Part model, mm, in its own coordinate system. A direction names the side the tool comes from. Round coordinates to 2 decimals unless told otherwise and drop trailing zeros. Loops run counter-clockwise (first coordinate to the right, second up) from the corner with the lowest first, then second, coordinate; pieces in that order, holes last.
1) Band-saw the part on A-A, the plane x = 0. Write the cut outline in (y, z), then the cut area to 3 significant figures.
2) Band-saw the part on B-B, the plane z = -1.5. Write the cut outline in (x, y), then the cut area to 3 significant figures.
3) Band-saw the part on C-C, the plane y = -17.25. Write the cut outline in (x, z), then the cut area to 3 significant figures.
4) 3-axis set-ups, long thin cutter, end or side, ignore diameter. For faces 1 (the flat face through (-21, 0, 15)), 2 (the cylindrical face through (-8.771, -12.325, 44.218)): which of +Z, -Z, +X, -X, +Y, -Y reach the whole face in a straight line?
5) Probe line 1 (Z direction, x = 0, y = -10.5); line 2 (X direction, y = -19, z = 29.5); line 3 (X direction, y = -18.25, z = 30). List the from-to ranges inside material, lowest first.
6) Drop flat-ended pins along their axis: P1, Ø6, axis at x = -23, y = -22.5, coming from the -Z side; P2, Ø10, axis at x = 24.94, z = 42.32, coming from the -Y side; P3, Ø1.5, axis at x = 19, z = 33, coming from the +Y side; P4, Ø2, axis at x = -32, y = -9, coming from the -Z side. Give the stop position or say it passes through.
from build123d import *

# Parameters (mm, degrees)
F0_R     = 5.194766
F0_R_2   = 8.44897
F0_R_3   = 5.580151
F1_DEPTH = 25


with BuildPart() as f1:
    # F0 (on Front) → F1 (new body)
    with BuildSketch(Plane.XZ):
        with BuildLine():
            ThreePointArc((-42.153431, 15.49969), (-22.537107, 7.573578), (-7.372486, -7.17965))
            ThreePointArc((-7.372486, -7.17965), (0.675671, -10.268612), (8.249685, -6.151716))
            Line((8.249685, -6.151716), (33.641666, 37.229096))
            ThreePointArc((33.641666, 37.229096), (34.332195, 45.988125), (27.889637, 51.962307))
            ThreePointArc((27.889637, 51.962307), (26.800193, 52.173359), (25.708755, 52.373848))
            ThreePointArc((25.708755, 52.373848), (-10.031283, 53.094379), (-44.25329, 42.76366))
            ThreePointArc((-44.25329, 42.76366), (-44.294203, 42.743895), (-44.335109, 42.724113))
            ThreePointArc((-44.335109, 42.724113), (-55.303805, 29.696455), (-45.187778, 15.996156))
            ThreePointArc((-45.187778, 15.996156), (-43.746778, 15.782133), (-42.311961, 15.529965))
            ThreePointArc((-42.311961, 15.529965), (-42.232685, 15.514886), (-42.153431, 15.49969))
        make_face()
        Circle(F0_R, mode=Mode.SUBTRACT)
        with Locations((-41.56223, 29.258074)):
            Circle(F0_R_2, mode=Mode.SUBTRACT)
        with BuildLine():
            Line((19.861759, 33.613489), (5.336992, 8.798718))
            ThreePointArc((5.336992, 8.798718), (0.233138, 10.288176), (-4.932946, 9.031443))
            ThreePointArc((-4.932946, 9.031443), (-15.984396, 17.984335), (-28.67212, 24.411659))
            ThreePointArc((-28.67212, 24.411659), (-27.982255, 31.544326), (-30.969534, 38.057929))
            ThreePointArc((-30.969534, 38.057929), (-8.443879, 44.251791), (14.867818, 42.724113))
            ThreePointArc((14.867818, 42.724113), (16.100782, 37.475942), (19.861759, 33.613489))
        make_face(mode=Mode.SUBTRACT)
        with Locations((24.941154, 42.321745)):
            Circle(F0_R_3, mode=Mode.SUBTRACT)
        with BuildLine():
            ThreePointArc((-44.25329, 42.76366), (-55.292646, 28.200564), (-42.153431, 15.49969))
            ThreePointArc((-42.153431, 15.49969), (-42.232685, 15.514886), (-42.311961, 15.529965))
            ThreePointArc((-42.311961, 15.529965), (-43.762253, 15.686672), (-45.187778, 15.996156))
            ThreePointArc((-45.187778, 15.996156), (-55.303805, 29.696455), (-44.335109, 42.724113))
            ThreePointArc((-44.335109, 42.724113), (-44.294203, 42.743895), (-44.25329, 42.76366))
        make_face()
        with BuildLine():
            ThreePointArc((25.708755, 52.373848), (26.800193, 52.173359), (27.889637, 51.962307))
            ThreePointArc((27.889637, 51.962307), (26.810555, 52.228274), (25.708755, 52.373848))
        make_face()
    extrude(amount=F1_DEPTH)


solid = f1.part
Reported:
1. outline: (-25, -10.29) - (0, -10.29) - (0, -5.19) - (-25, -5.19) - close; (-25, 5.19) - (0, 5.19) - (0, 10.29) - (-25, 10.29) - close; (-25, 44.6) - (0, 44.6) - (0, 54.03) - (-25, 54.03) - close
1. area: 490 mm2
2. outline: (-11.89, -25) - (-4.97, -25) - (-4.97, 0) - (-11.89, 0) - close; (4.97, -25) - (10.97, -25) - (10.97, 0) - (4.97, 0) - close
2. area: 323 mm2
3. outline: (-44.25, 42.76) arc R13.77 ccw to (-42.15, 15.5) arc R54.92 cw to (-7.37, -7.18) arc R10.29 ccw to (8.25, -6.15) - (33.64, 37.23) arc R10.08 ccw to (27.89, 51.96) arc R10.08 ccw to (25.71, 52.37) arc R114.56 ccw to start; hole circle Ø16.9 at (-41.56, 29.26); hole (-45.19, 16) arc R13.75 ccw to (-42.31, 15.53) arc R54.92 ccw to start; hole (-30.97, 38.06) arc R13.77 cw to (-28.67, 24.41) arc R67.22 cw to (-4.93, 9.03) arc R10.29 cw to (5.34, 8.8) - (19.86, 33.61) arc R10.08 cw to (14.87, 42.72) arc R70.32 ccw to start; hole circle Ø10.39 at (0, 0); hole circle Ø11.16 at (24.94, 42.32)
3. area: 2,050 mm2
4. face 1: +Z, -Z, +X, -X, +Y
4. face 2: +Y, -Y
5. line 1: z = -10.29 to -5.19, 5.19 to 10.29, 44.6 to 54.03
5. line 2: x = -55.33 to -50.01, -33.12 to -27.79, 17.45 to 29.12
5. line 3: x = -55.31 to -49.98, -33.15 to -27.81, 17.75 to 29.41
6. P1: stops at z = 5.82
6. P2: passes through
6. P3: stops at y = 0
6. P4: stops at z = 12.09
